Build history of the part. All positions in model axes, mm. A direction names the side the tool comes from. Give positions to 0.01 mm unless a question says otherwise; leave off trailing zeros. Order: outer loops, then holes, each group sorted by start corner. A loop starts at its lowest first (then second) coordinate and runs counter-clockwise, first axis right, second up. Notation, with made-up numbers: (1, 13.5) - (24, 13.5) arc R26 cw to (24, 42.5) - close; hole circle Ø6 at (48, 57.5). An arc over 180 degrees is marked (long way). Use a Markdown table: item, result.
from build123d import *

# Parameters (mm, degrees)
SKETCH1_W           = 14
SKETCH1_H           = 26
BOSS_EXTRUDE1_DEPTH = 2.5
SKETCH2_W           = 17
SKETCH2_H           = 28
BOSS_EXTRUDE2_DEPTH = 1.6
SKETCH3_W           = 9
SKETCH3_H           = 7.4
BOSS_EXTRUDE3_DEPTH = 3.2
SKETCH4_W           = 5
SKETCH4_H           = 5
BOSS_EXTRUDE4_DEPTH = 1.5
SKETCH5_W           = 3
SKETCH5_H           = 3
BOSS_EXTRUDE5_DEPTH = 1.2
SKETCH6_W           = 4
SKETCH6_H           = 3
BOSS_EXTRUDE6_DEPTH = 1.2


with BuildPart() as part:
    # Sketch1 → Boss-Extrude1 (new body)
    with BuildSketch(Plane.XY.offset(10.6)):
        with Locations((18, 36)):
            Rectangle(SKETCH1_W, SKETCH1_H)
    extrude(amount=BOSS_EXTRUDE1_DEPTH)

    # Sketch2 → Boss-Extrude2 (add)
    with BuildSketch(Plane.XY.offset(13.1)):
        with Locations((18, 36)):
            Rectangle(SKETCH2_W, SKETCH2_H)
    extrude(amount=BOSS_EXTRUDE2_DEPTH)

    # Sketch3 → Boss-Extrude3 (add)
    with BuildSketch(Plane.XY.offset(14.7)):
        with Locations((18, 24.9)):
            Rectangle(SKETCH3_W, SKETCH3_H)
    extrude(amount=BOSS_EXTRUDE3_DEPTH)

    # Sketch4 → Boss-Extrude4 (add)
    with BuildSketch(Plane.XY.offset(14.7)):
        with Locations((18, 36.5)):
            Rectangle(SKETCH4_W, SKETCH4_H)
    extrude(amount=BOSS_EXTRUDE4_DEPTH)

    # Sketch5 → Boss-Extrude5 (add)
    with BuildSketch(Plane.XY.offset(14.7)):
        with Locations((18, 43.5)):
            Rectangle(SKETCH5_W, SKETCH5_H)
    extrude(amount=BOSS_EXTRUDE5_DEPTH)

    # Sketch6 → Boss-Extrude6 (add)
    with BuildSketch(Plane.XY.offset(14.7)):
        with Locations((18, 47.5)):
            Rectangle(SKETCH6_W, SKETCH6_H)
    extrude(amount=BOSS_EXTRUDE6_DEPTH)


solid = part.part
1) Slice it at D-D (y = 47). Write the cut outline in (x, z).
Computed:
| item | result |
|---|---|
| outline | (9.5, 13.1) - (11, 13.1) - (11, 10.6) - (25, 10.6) - (25, 13.1) - (26.5, 13.1) - (26.5, 14.7) - (20, 14.7) - (20, 15.9) - (16, 15.9) - (16, 14.7) - (9.5, 14.7) - close |
2) Pin check, flat tips, straight feed: P1, Ø1.2, axis at x = 20, z = 12, coming from the -Y side; P2, Ø0.9, axis at x = 20, y = 22, coming from the -Z side; P3, Ø1.2, axis at y = 35.5, z = 15.5, coming from the +X side; P4, Ø3, axis at x = 16.5, z = 12, coming from the +Y side. Stop position of each tip, or through.
Computed:
| item | result |
|---|---|
| P1 | stops at y = 23 |
| P2 | stops at z = 13.1 |
| P3 | stops at x = 20.5 |
| P4 | stops at y = 50 |
3) Slice it at B-B (y = 32.25). Write the cut outline in (x, z).
Computed:
| item | result |
|---|---|
| outline | (9.5, 13.1) - (11, 13.1) - (11, 10.6) - (25, 10.6) - (25, 13.1) - (26.5, 13.1) - (26.5, 14.7) - (9.5, 14.7) - close |
4) Two-plate mould, pull along Y, no slides. Class faces 1 (the flat face through (13.5, 25, 16)), 2 (the flat face through (18, 49, 15)), 3 (the flat face through (16.5, 43, 15)): +Y half, -Y half, draft (parallel to the pull), parting line (faces both ways), or undercut.
Computed:
| item | result |
|---|---|
| face 1 | draft |
| face 2 | +Y half |
| face 3 | undercut |
5) Wall check: line 1 (Z direction, x = 19, y = 30); line 2 (X direction, y = 25.5, z = 17); line 3 (Y direction, x = 16.5, z = 11.25). Give the ranges that are in metal, low to high. Write a range as from..to.
Computed:
| item | result |
|---|---|
| line 1 | z = 10.6..14.7 |
| line 2 | x = 13.5..22.5 |
| line 3 | y = 23..49 |
6) Slice it at A-A (z = 15.25). Write the cut outline in (x, y).
Computed:
| item | result |
|---|---|
| outline | (13.5, 21.2) - (22.5, 21.2) - (22.5, 28.6) - (13.5, 28.6) - close; (15.5, 34) - (20.5, 34) - (20.5, 39) - (15.5, 39) - close; (16, 46) - (20, 46) - (20, 49) - (16, 49) - close; (16.5, 42) - (19.5, 42) - (19.5, 45) - (16.5, 45) - close |
7) Slice it at C-C (x = 14.25). Write the cut outline in (y, z).
Computed:
| item | result |
|---|---|
| outline | (21.2, 14.7) - (22, 14.7) - (22, 13.1) - (23, 13.1) - (23, 10.6) - (49, 10.6) - (49, 13.1) - (50, 13.1) - (50, 14.7) - (28.6, 14.7) - (28.6, 17.9) - (21.2, 17.9) - close |
8) Tool access for faces 4 (the flat face through (20, 47, 15)), 5 (the flat face through (25, 36, 12)), 6 (the flat face through (18, 37, 16.2)), 7 (the flat face through (16, 47, 15)): list every direction of +Z, -Z, +X, -X, +Y, -Y with a clear straight run to the whole face (end or side of a thin tool).
Computed:
| item | result |
|---|---|
| face 4 | +Z, +X, +Y |
| face 5 | -Z, +X, +Y, -Y |
| face 6 | +Z, +X, -X, +Y |
| face 7 | +Z, -X, +Y |
